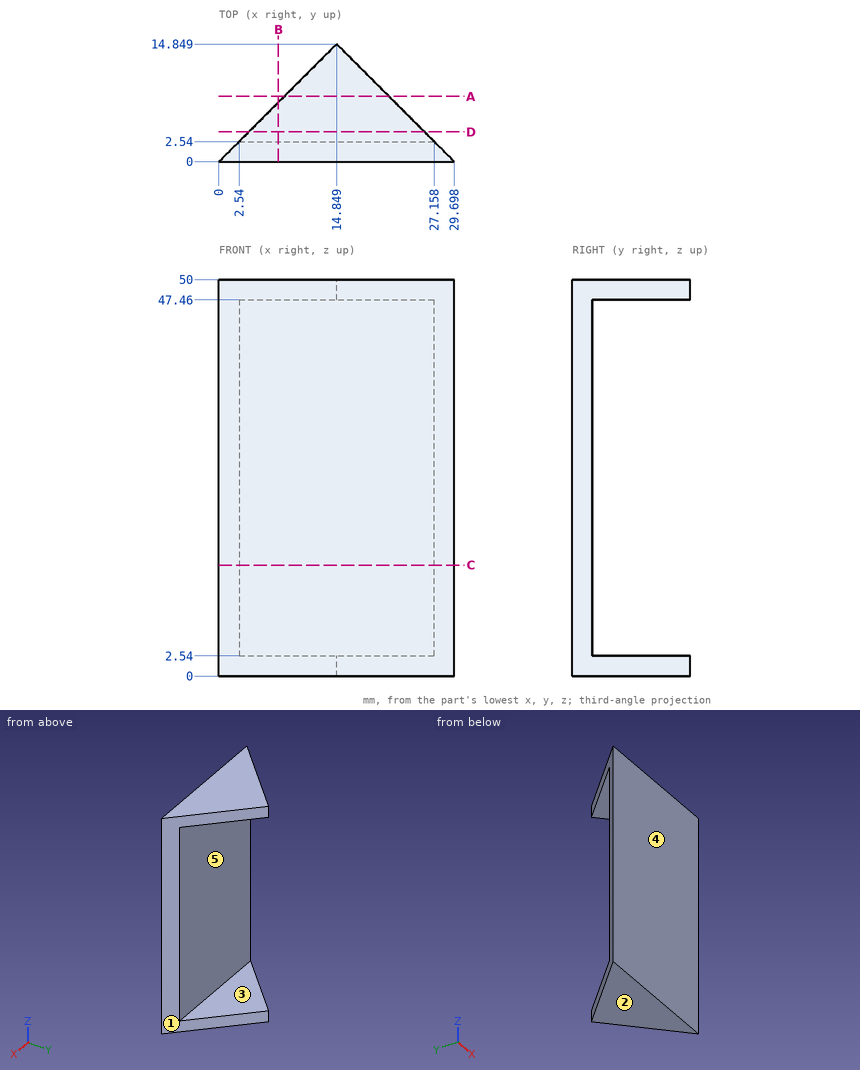
Here's the drawing with two shaded views (mm, measured from the low corner). I have some questions. A direction names the side the tool comes from. Coordinates: 2 decimals unless noted, no trailing zeros. Loops run counter-clockwise (first coordinate to the right, second up) from the corner with the lowest first, then second, coordinate; pieces in that order, holes last. Notation, with made-up numbers: (76.25, -1.75) -> (101.25, -1.75) arc R30 cw to (101.25, 22.25) -> close; hole circle Ø3 at (-9, 2.25). An arc over 180 degrees is marked (long way). Answer in a Markdown table with one row per item.
(1) For the marked faces 4 and 5, which set-ups out of +Z, -Z, +X, -X, +Y, -Y let a thin tool reach every point of the face, with its end or its side?
Results found:
| item | result |
|---|---|
| face 4 | +Z, -Z, +X, -X, -Y |
| face 5 | +X, -X, +Y |
(2) Imagine slicing it at D-D (y = 3.75). List the corners of the cut face in (x, z) for me.
Results found:
| item | result |
|---|---|
| outline | (3.75, 0) -> (25.95, 0) -> (25.95, 2.54) -> (3.75, 2.54) -> close; (3.75, 47.46) -> (25.95, 47.46) -> (25.95, 50) -> (3.75, 50) -> close |
(3) Thinking about a two-plate mould opening in Z: for the marked faces 1, 2 and 3, which applies, released by +Z, released by -Z, zero draft, split by the parting line, or undercut?
Results found:
| item | result |
|---|---|
| face 1 | zero draft |
| face 2 | released by -Z |
| face 3 | undercut |
(4) Imagine slicing it at A-A (y = 8.25). List the corners of the cut face in (x, z) for me.
Results found:
| item | result |
|---|---|
| outline | (8.25, 0) -> (21.45, 0) -> (21.45, 2.54) -> (8.25, 2.54) -> close; (8.25, 47.46) -> (21.45, 47.46) -> (21.45, 50) -> (8.25, 50) -> close |
(5) Imagine slicing it at C-C (z = 14). List the corners of the cut face in (x, y) for me.
Results found:
| item | result |
|---|---|
| outline | (0, 0) -> (29.7, 0) -> (27.16, 2.54) -> (2.54, 2.54) -> close |
(6) Imagine slicing it at B-B (x = 7.5). List the corners of the cut face in (y, z) for me.
Results found:
| item | result |
|---|---|
| outline | (0, 0) -> (7.5, 0) -> (7.5, 2.54) -> (2.54, 2.54) -> (2.54, 47.46) -> (7.5, 47.46) -> (7.5, 50) -> (0, 50) -> close |
(7) Will these pins go through, and if not, where does the flat tip stop? pin 1 Ø10 at (x, z) = (10, 29.5) entering from +Y; pin 2 Ø3.5 at (x, y) = (8.5, 11.5) entering from -Z.
Results found:
| item | result |
|---|---|
| pin 1 | stops at y = 2.54 |
| pin 2 | passes through |
(8) If I drill on probe 1 along Z at (x, y) = (18.25, 6.5); probe 2 along Y at (x, z) = (18, 12); probe 3 along Y at (x, z) = (20.5, 47.5), over which ranges is the centre line in solid material (lowest first)?
Results found:
| item | result |
|---|---|
| probe 1 | z = 0 to 2.54, 47.46 to 50 |
| probe 2 | y = 0 to 2.54 |
| probe 3 | y = 0 to 9.2 |
